The model under review builds one solid part; all positions refer to its coordinate system, in mm. Face numbers are marked on the shaded views. A direction names the side the tool comes from. Coordinates: 2 decimals unless noted, no trailing zeros. Write each loop counter-clockwise with the first axis right and the second up, starting at its lowest first coordinate (ties: lowest second). Pieces come first, ordered by that corner, then holes.
```python
from build123d import *

# Parameters (mm, degrees)
PAD006_DEPTH            = 11.5
THICKNESS001_T          = -1
POCKET002_DEPTH         = 5
BODY017_PLACEMENT_ANGLE = 180


with BuildPart() as part:
    # Sketch008 → Pad006 (new body)
    with BuildSketch(Plane.XY):
        Polygon((-20.497056, 69.8), (20.497056, 69.8), (40.5, 49.797056), (40.5, 8.802944), (31.697056, 0), (40.5, -8.802944), (40.5, -49.797056), (20.497056, -69.8), (-20.497056, -69.8), (-40.5, -49.797056), (-40.5, -8.802944), (-31.697056, 0), (-40.5, 8.802944), (-40.5, 49.797056), align=None)
    extrude(amount=PAD006_DEPTH)

    # Thickness001
    thickness001_openings = [part.faces().sort_by_distance(p)[0] for p in [
        (0, 0, 11.5),
    ]]
    offset(amount=THICKNESS001_T, openings=thickness001_openings)

    # Sketch009 (on Face33 of Thickness001) → Pocket002 (cut)
    with BuildSketch(Plane.XY.offset(1)):
        Polygon((-18.840202, 65.8), (18.840202, 65.8), (36.5, 48.140202), (36.5, 10.459798), (26.040202, 0), (36.5, -10.459798), (36.5, -48.140202), (18.840202, -65.8), (-18.840202, -65.8), (-36.5, -48.140202), (-36.5, -10.459798), (-26.040202, 0), (-36.5, 10.459798), (-36.5, 48.140202), align=None)
    extrude(amount=-POCKET002_DEPTH, mode=Mode.SUBTRACT)


with BuildPart() as part_1:
    # Body017 placement: moved
    add(part.part.moved(Location((0, 0, 19))).rotate(Axis((0, 0, 19), (0, 1, 0)), BODY017_PLACEMENT_ANGLE))


solid = part_1.part
```
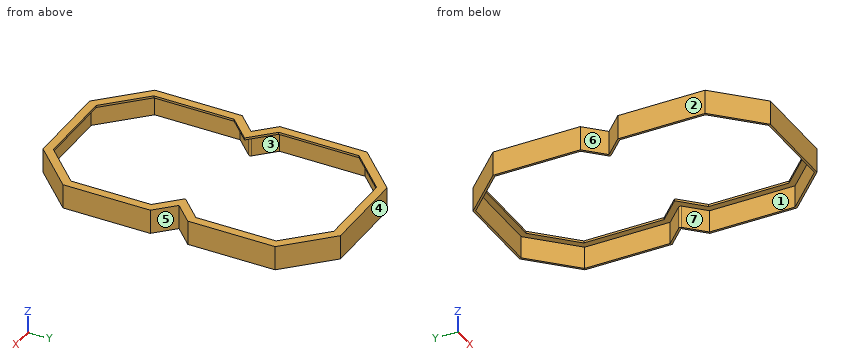
Item 1: Take a section at D-D, the plane x = 27.5. Write out the cut boundary in (y, z), plus the area to 3 significant figures.
Solved:
outline: (-62.8, 7.5) - (-61.38, 7.5) - (-61.38, 18) - (-57.14, 18) - (-57.14, 19) - (-62.8, 19) - close; (-1.46, 18) - (1.46, 18) - (1.46, 19) - (-1.46, 19) - close; (57.14, 18) - (61.38, 18) - (61.38, 7.5) - (62.8, 7.5) - (62.8, 19) - (57.14, 19) - close
area: 43.9 mm2
Item 2: Mouldability with a two-part tool opening along Y and no side actions: class the marked faces 1, 2, 3 and 4 as pulls with the +Y half, pulls with the -Y half, needs draft (parallel to the pull), parting line crosses it, or undercut.
Solved:
face 1: undercut
face 2: needs draft
face 3: undercut
face 4: pulls with the +Y half
Item 3: Take a section at B-B, the plane x = 3.5. Write out the cut boundary in (y, z), plus the area to 3 significant figures.
Solved:
outline: (-69.8, 7.5) - (-68.8, 7.5) - (-68.8, 18) - (-65.8, 18) - (-65.8, 19) - (-69.8, 19) - close; (65.8, 18) - (68.8, 18) - (68.8, 7.5) - (69.8, 7.5) - (69.8, 19) - (65.8, 19) - close
area: 29.0 mm2
Item 4: Machinability: for the marked faces 5, 6 and 7, which of the approach directions +Z, -Z, +X, -X, +Y, -Y give a long, thin tool a straight path to every point of the face, cutting with its end or side? Answer none if there is none.
Solved:
face 5: +Z, -Z, +X
face 6: +Z, -Z, -X
face 7: -Z
Item 5: Take a section at A-A, the plane y = -34. Write out the cut boundary in (x, z).
Solved:
outline: (-40.5, 7.5) - (-39.5, 7.5) - (-39.5, 18) - (-36.5, 18) - (-36.5, 19) - (-40.5, 19) - close; (36.5, 18) - (39.5, 18) - (39.5, 7.5) - (40.5, 7.5) - (40.5, 19) - (36.5, 19) - close
Item 6: For pin 1 (1.5 mm diameter, centred on x = 24.5, z = 9.5, fed in from -Y); pin 2 (1.5 mm diameter, centred on x = 23.5, z = 17.5, fed in from -Y); pin 3 (4 mm diameter, centred on x = -24.5, z = 10, fed in from -Y), all flat-tipped, find the tip position at first contact; note any pin that passes through.
Solved:
pin 1: stops at y = -66.55
pin 2: stops at y = -67.55
pin 3: stops at y = -67.8
Item 7: To check wall thickness, follow line 1 along Y through (x, z) = (2.5, 8.5); line 2 along Y through (x, z) = (-36.5, 15); line 3 along X through (y, z) = (20, 13.5). State the ranges of each line that lie inside material, in increasing order.
Solved:
line 1: y = -69.8 to -68.8, 68.8 to 69.8
line 2: y = -53.8 to -52.38, -6.22 to -4.8, 4.8 to 6.22, 52.38 to 53.8
line 3: x = -40.5 to -39.5, 39.5 to 40.5
